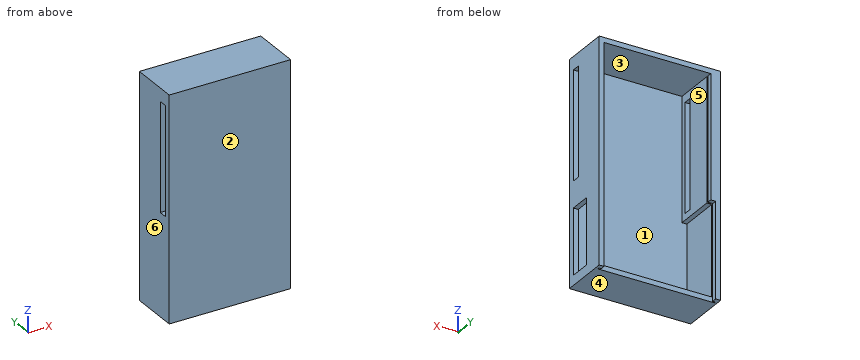
Autodesk Inventor part; units mm, degrees
ref_plane "Work Plane1" through (-34, 30, -130) normal (-1, 0, 0) x (0, 0, 1)
ref_plane "Work Plane2" through (0, 30, -65) normal (0, 0, -1) x (-1, 0, 0)
ref_plane "Work Plane3" through (-34, 30, -75) normal (1, 0, 0) x (0, 0, -1)
sketch "Sketch1" plane through (0, 0, 0) normal (0, 1, 0) x (-1, 0, 0)
  line L0 (0, 0) -> (68, 0)
  line L1 (68, -75) -> (68, -130)
  line L2 (68, -130) -> (0, -130)
  line L3 (0, -130) -> (0, 0)
  line L4 (68, 0) -> (65, 0)
  line L5 (65, 0) -> (65, -75)
  line L6 (65, -75) -> (68, -75)
  line L7 (0, 0) -> (0, 1)
  line L8 (0, 1) -> (69, 1)
  line L9 (69, 1) -> (69, -131)
  line L10 (69, -131) -> (-1, -131)
  line L11 (-1, -131) -> (-1, 1)
  line L12 (-1, 1) -> (0, 1)
  dimension "d0" = 68
  dimension "d1" = 130
  dimension "d2" = 3
  dimension "d3" = 75
  dimension "d4" = 1
  dimension "d5" = 69
  dimension "d6" = 132
  dimension "d7" = 70
extrude "Extrusion1" add sketch "Sketch1" along normal blind 30
sketch "Sketch2" plane through (0, 0, 0) normal (0, -1, 0) x (1, 0, 0)
  line L0 (0, 0) -> (-65, 0)
  line L1 (-68, -75) -> (-68, -130)
  line L2 (0, 0) -> (-68, 0)
  line L3 (-68, 0) -> (-68, -130)
  line L4 (-68, -130) -> (0, -130)
  line L5 (0, -130) -> (0, 0)
extrude "Extrusion2" add sketch "Sketch2" against normal blind 1
sketch "Sketch3" plane through (1, 0, 1) normal (1, 0, 0) x (0, 0, -1)
  line L0 (131, 1) -> (1, 1)
  line L1 (1, 1) -> (1, 6)
  line L2 (1, 1) -> (1, 30)
  line L3 (1, 6) -> (1, 1)
  line L4 (1, 6) -> (6, 6)
  line L5 (6, 9.0023) -> (72, 9.0023)
  line L6 (72, 9.0023) -> (72, 4.0023)
  line L7 (72, 4.0023) -> (6, 4.0023)
  line L8 (6, 4.0023) -> (6, 9.0023)
  line L9 (6, 1) -> (6, 4)
  point P0 (1, 0)
  dimension "d12" = 5
  dimension "d13" = 5
  dimension "d14" = 5
  dimension "d15" = 66
  dimension "d23" = 3
extrude "Extrusion3" cut sketch "Sketch3" along normal blind 34.75 and the other way blind 4
ref_plane "Work Plane1" through (-34, 30, -130) normal (-1, 0, 0) x (0, 0, 1)
mirror "Mirror1" about plane through (-34, 30, -130) normal (-1, 0, 0) of "Extrusion3"
sketch "Sketch4" plane through (1, 0, 1) normal (1, 0, 0) x (0, 0, -1)
  line L0 (131, 1) -> (131, 30)
  line L1 (131, 1) -> (128, 1)
  line L2 (76, 1) -> (131, 1)
  line L3 (128, 3.992) -> (128, 16.992)
  line L4 (128, 16.992) -> (88, 16.992)
  line L5 (88, 16.992) -> (88, 3.992)
  line L6 (88, 3.992) -> (128, 3.992)
  line L7 (132, 0) -> (0, 0)
  line L8 (88, 1) -> (88, 4)
  point P0 (1, 0)
  dimension "d18" = 3
  dimension "d19" = 13
  dimension "d20" = 40
  dimension "d24" = 3
extrude "Extrusion4" cut sketch "Sketch4" against normal blind 5
sketch "Sketch5" plane through (-69, 0, 1) normal (0, 0, 1) x (1, 0, 0)
  line L0 (70, 0) -> (70, 30)
  line L1 (0, 0) -> (70, 0)
  line L2 (70, 0) -> (70, 30)
  line L3 (70, 30) -> (0, 30)
  line L4 (0, 30) -> (0, 0)
  point P0 (69, 0)
extrude "Extrusion5" add sketch "Sketch5" along normal blind 2
ref_plane "Work Plane2" through (0, 30, -65) normal (0, 0, -1) x (-1, 0, 0)
mirror "Mirror2" about plane through (0, 30, -65) normal (0, 0, -1) of "Extrusion5"
sketch "Sketch6" plane through (1, 0, 3) normal (1, 0, 0) x (0, 0, -1)
  line L0 (0, 0) -> (0, 30)
  line L1 (0, 0) -> (136, 0)
  line L2 (0, 30) -> (136, 30)
  line L3 (136, 30) -> (136, 0)
  line L4 (136, 0) -> (0, 0)
  line L5 (0, 0) -> (0, 30)
  point P0 (3, 0)
extrude "Extrusion6" add sketch "Sketch6" along normal blind 2
ref_plane "Work Plane3" through (-34, 30, -75) normal (1, 0, 0) x (0, 0, -1)
mirror "Mirror3" about plane through (-34, 30, -75) normal (1, 0, 0) of "Extrusion6"
sketch "Sketch7" plane through (-71, 0, -133) normal (-1, 0, 0) x (0, 0, 1)
  line L0 (62, 9.0023) -> (128, 9.0023)
  line L1 (128, 4.0023) -> (62, 4.0023)
  line L2 (62, 9.0023) -> (128, 9.0023)
  line L3 (128, 9.0023) -> (128, 4.0023)
  line L4 (128, 4.0023) -> (62, 4.0023)
  line L5 (62, 4.0023) -> (62, 9.0023)
  point P0 (133, 0)
  point P1 (62, 4.0023)
extrude "Extrusion7" cut sketch "Sketch7" against normal blind 34.75
mirror "Mirror4" about plane through (-34, 30, -130) normal (-1, 0, 0) of "Extrusion7"
sketch "Sketch8" plane through (3, 0, 3) normal (1, 0, 0) x (0, 0, -1)
  line L0 (130, 16.992) -> (90, 16.992)
  line L1 (90, 3.992) -> (130, 3.992)
  line L2 (90, 16.992) -> (130, 16.992)
  line L3 (130, 16.992) -> (130, 3.992)
  line L4 (130, 3.992) -> (90, 3.992)
  line L5 (90, 3.992) -> (90, 16.992)
  point P0 (3, 0)
extrude "Extrusion8" cut sketch "Sketch8" against normal blind 34.75
sketch "Sketch9" plane through (3, 0, -133) normal (0, 0, -1) x (-1, 0, 0)
  line L0 (71, 1) -> (71, 30)
  line L1 (71, 30) -> (71, 27)
  line L2 (71, 1) -> (71, 30)
  line L3 (71, 27) -> (72.5, 27)
  line L4 (74, 0) -> (74, 30)
  line L5 (74, 30) -> (0, 30)
  line L6 (3, 30) -> (3, 27)
  line L7 (3, 27) -> (1.5, 27)
  line L8 (72.5, 27) -> (1.5, 27)
  line L9 (1.5, 27) -> (1.5, 26)
  line L10 (1.5, 26) -> (72.5, 26)
  line L11 (72.5, 26) -> (72.5, 27)
  point P0 (3, 0)
  dimension "d35" = 3
  dimension "d36" = 1.5
  dimension "d37" = 1.5
  dimension "d38" = 1
extrude "Extrusion9" cut sketch "Sketch9" against normal blind 133 contours L3 L11 L10 L0 | L0 L10 L9 L7 L8
sketch "Sketch10" plane through (3, 0, -133) normal (0, 0, -1) x (-1, 0, 0)
  line L0 (0, 30) -> (74, 30)
  line L1 (71, 27) -> (3, 27)
  line L2 (3, 30) -> (71, 30)
  line L3 (71, 30) -> (71, 27)
  line L4 (71, 27) -> (3, 27)
  line L5 (3, 27) -> (3, 30)
  point P0 (3, 0)
extrude "Extrusion10" cut sketch "Sketch10" against normal blind 3
properties part number "ESP 32 a&b gabung test 4"
Verification items for the finished model (mm, model axes). Face numbers are marked on the shaded views. A direction names the side the tool comes from. Coordinates: 2 decimals unless noted, no trailing zeros. Loops run counter-clockwise (first coordinate to the right, second up) from the corner with the lowest first, then second, coordinate; pieces in that order, holes last. Notation, with made-up numbers: (43.5, 47.25) -> (60.5, 47.25) arc R33 ccw to (60.5, 85.25) -> close; hole circle Ø3 at (36, 5). An arc over 180 degrees is marked (long way). Answer as a JSON object with one key per item and string values. Group by question number.
Item 1: Tool access check on the marked faces 5 and 6. Record the directions out of +Z, -Z, +X, -X, +Y, -Y that give a thin tool (end or side, any length) a straight path to the whole face; none if there is none.
Item 2: Sectioned sample at C-C on z = -90.5. Record the boundary of the cut face in (x, y).
Item 3: Mould release check, pull along Z, two halves, no side actions. Record for the marked faces 1, 2, 3 and 4: +Z half, -Z half, draft (parallel to the pull), parting line (faces both ways), or undercut.
Item 4: Depth check by flat-ended pin: pin 1 (6 mm diameter, centred on x = -33, z = -75.5, fed in from +Y); pin 2 (1 mm diameter, centred on y = 8, z = -12, fed in from -X). Enter the tip coordinate at first touch or a pass-through.
Item 5: Scan lines: probe 1 along Z at (x, y) = (-57, 14.75); probe 2 along X at (y, z) = (22.25, -50); probe 3 along X at (y, z) = (2.5, -125.5). Record each from-to range of solid material in increasing order.
Item 6: Sectioned sample at B-B on z = -14. Record the boundary of the cut face in (x, y).
Item 7: Sectioned sample at A-A on y = 6. Record the boundary of the cut face in (x, z), plus the area to 3 significant figures.
Item 8: Sectioned sample at D-D on x = -62. Record the boundary of the cut face in (y, z), plus the area to 3 significant figures.
Evaluation:
{
 "1": {"face 5": "+Y", "face 6": "+Z, -Z, -X, +Y, -Y"},
 "2": {"outline": "(-71, 0) -> (3, 0) -> (3, 3.99) -> (0, 3.99) -> (0, 1) -> (-68, 1) -> (-68, 26) -> (-69.5, 26) -> (-69.5, 27) -> (-68, 27) -> (-68, 30) -> (-71, 30) -> close; (0, 16.99) -> (3, 16.99) -> (3, 30) -> (0, 30) -> (0, 27) -> (1.5, 27) -> (1.5, 26) -> (0, 26) -> close"},
 "3": {"face 1": "undercut", "face 2": "draft", "face 3": "undercut", "face 4": "-Z half"},
 "4": {"pin 1": "stops at y = 1", "pin 2": "passes through"},
 "5": {"probe 1": "z = -133 to -130, 0 to 3", "probe 2": "x = -71 to -65, 0 to 3", "probe 3": "x = -71 to -68, 0 to 3"},
 "6": {"outline": "(-71, 0) -> (3, 0) -> (3, 4) -> (0, 4) -> (0, 1) -> (-65, 1) -> (-65, 4) -> (-71, 4) -> close; (-71, 9) -> (-65, 9) -> (-65, 26) -> (-69.5, 26) -> (-69.5, 27) -> (-65, 27) -> (-65, 30) -> (-71, 30) -> close; (0, 9) -> (3, 9) -> (3, 30) -> (0, 30) -> (0, 27) -> (1.5, 27) -> (1.5, 26) -> (0, 26) -> close"},
 "7": {"outline": "(-71, -133) -> (3, -133) -> (3, -127) -> (0, -127) -> (0, -130) -> (-68, -130) -> (-68, -75) -> (-65, -75) -> (-65, -71) -> (-71, -71) -> close; (-71, -5) -> (-65, -5) -> (-65, 0) -> (0, 0) -> (0, -5) -> (3, -5) -> (3, 3) -> (-71, 3) -> close; (0, -87) -> (3, -87) -> (3, -71) -> (0, -71) -> close", "area": "735 mm²"},
 "8": {"outline": "(0, -133) -> (26, -133) -> (26, -130) -> (1, -130) -> (1, 0) -> (30, 0) -> (30, 3) -> (0, 3) -> close", "area": "298 mm²"}
}
